Check sheet for the modelled part. Datum: model origin and axes. Units: mm. A direction names the side the tool comes from. Give positions to 0.01 mm unless a question says otherwise; leave off trailing zeros. Order: outer loops, then holes, each group sorted by start corner. A loop starts at its lowest first (then second) coordinate and runs counter-clockwise, first axis right, second up.
```python
from build123d import *

# Parameters (mm, degrees)
BOSS_EXTRUDE1_DEPTH     = 5.3
CIRPATTERN1_COUNT       = 10
FILLET1_R               = 0.2
FILLET3_R               = 0.2
SKETCH2_R               = 10
SKETCH2_R_2             = 4.05
BOSS_EXTRUDE2_DEPTH     = 16.7
CUT_EXTRUDE1_DEPTH      = 29.341701561
CUT_EXTRUDE1_DEPTH_BACK = 29.341701561
SKETCH2_2_R             = 4.05


with BuildPart() as part:
    # Sketch1 → Boss-Extrude1 (new body)
    with BuildSketch(Plane(origin=(0, 0, 0), x_dir=(0, 0, -1), z_dir=(1, 0, 0))):
        with BuildLine():
            Line((0, 0), (0, 16.75))
            Line((0, 16.75), (1.800167381, 14.035023954))
            ThreePointArc((1.800167381, 14.035023954), (3.754556482, 11.555336673), (6.793214092, 12.412684734))
            Line((6.793214092, 12.412684734), (9.845402976, 13.551034656))
            Line((9.845402976, 13.551034656), (0, 0))
        make_face()
    boss_extrude1 = extrude(amount=BOSS_EXTRUDE1_DEPTH)

    # CirPattern1: Boss-Extrude1 ×10 about axis
    cirpattern1_axis = Axis((0, 0, 0), (1, 0, 0))
    for i in range(1, CIRPATTERN1_COUNT):
        add(boss_extrude1.rotate(cirpattern1_axis, i * 360 / CIRPATTERN1_COUNT))

    # Fillet1
    fillet1_edges = [part.edges().sort_by_distance(p)[0] for p in [
        (2.65, 16.75, 0),
    ]]
    fillet(fillet1_edges, radius=FILLET1_R)

    # Fillet3
    fillet3_edges = [part.edges().sort_by_distance(p)[0] for p in [
        (2.65, 13.551034656, -9.845402976),
        (2.65, 13.551034656, 9.845402976),
        (2.65, 5.176034656, 15.930196648),
        (2.65, -5.176034656, 15.930196648),
        (2.65, -13.551034656, 9.845402976),
        (2.65, -16.75, 0),
        (2.65, -13.551034656, -9.845402976),
        (2.65, -5.176034656, -15.930196648),
        (2.65, 5.176034656, -15.930196648),
    ]]
    fillet(fillet3_edges, radius=FILLET3_R)

    # Sketch2 → Boss-Extrude2 (add)
    with BuildSketch(Plane.ZY):
        with Locations(Location((0, 0, 0), (0, 0, 180))):
            Circle(SKETCH2_R)
        Circle(SKETCH2_R_2, mode=Mode.SUBTRACT)
    extrude(amount=BOSS_EXTRUDE2_DEPTH)

    # Sketch2_2 → Cut-Extrude1 (cut, two sides: drawn at the far end of the back side and taken through both)
    with BuildSketch(Plane.ZY.offset(-CUT_EXTRUDE1_DEPTH_BACK)):
        Circle(SKETCH2_2_R)
    extrude(amount=CUT_EXTRUDE1_DEPTH + CUT_EXTRUDE1_DEPTH_BACK, mode=Mode.SUBTRACT)


solid = part.part
```
(1) Sectioned sample at B-B (z = -1). Enter the section's corners in (x, y).
(2) Thickness scan on L1, parallel to Y at x = -3, z = 0; L2, parallel to X at y = 6, z = 8.5; L3, parallel to Y at x = -15, z = 2. Record the ranges inside material, lowest first.
(3) Go/stop test with flat-tipped pins: P1, Ø2, axis at x = -13.5, y = -7, coming from the +Z side; P2, Ø12, axis at x = -7, y = 12, coming from the -Z side; P3, Ø4, axis at x = -9, z = -3, coming from the -Y side. Record where each tip stops, or that it passes through.
(4) Sectioned sample at A-A (y = 0). Enter the section's corners in (x, z), plus the area to 3 significant figures.
(5) Release check for a two-part mould opening along Y. For faces 1 (the face through (2.613, 12.922, -8.159)), 2 (the face through (2.613, -3.766, -14.811)), 3 (the face through (-16.7, -0.1, -4.3)) record: released by +Y, released by -Y, zero draft, split by the parting line, or undercut.
(6) Tool access check on faces 4 (the face through (2.613, 12.936, 8.197)), 5 (the face through (0, 2, -10)), 6 (the face through (2.61, -11.79, 9.77)), 7 (the face through (2.61, -11.75, -9.77)). Record the directions out of +Z, -Z, +X, -X, +Y, -Y that give a thin tool (end or side, any length) a straight path to the whole face; none if there is none.
(7) Sectioned sample at C-C (y = -12). Enter the section's corners in (x, z).
(8) Sectioned sample at D-D (x = -2.75). Enter the section's corners in (y, z).
Values follow:
1. outline: (-16.7, -9.95) - (0, -9.95) - (0, -15.24) - (5.3, -15.24) - (5.3, -3.92) - (-16.7, -3.92) - close; (-16.7, 3.92) - (5.3, 3.92) - (5.3, 15.24) - (0, 15.24) - (0, 9.95) - (-16.7, 9.95) - close
2. L1: y = -10 to -4.05, 4.05 to 10
2. L2: x = 0 to 5.3
2. L3: y = -9.8 to -3.52, 3.52 to 9.8
3. P1: stops at z = 8
3. P2: stops at z = -8
3. P3: stops at y = -9.95
4. outline: (-16.7, -10) - (0, -10) - (0, -12.15) - (5.3, -12.15) - (5.3, -4.05) - (-16.7, -4.05) - close; (-16.7, 4.05) - (5.3, 4.05) - (5.3, 12.15) - (0, 12.15) - (0, 10) - (-16.7, 10) - close
4. area: 285 mm2
5. face 1: released by +Y
5. face 2: undercut
5. face 3: zero draft
6. face 4: +X, -X, +Y
6. face 5: -X
6. face 6: +Z, +X, -X
6. face 7: -Z, +X, -X
7. outline: (0, -9.78) - (5.3, -9.78) - (5.3, -6.36) - (0, -6.36) - close; (0, -2.91) - (5.3, -2.91) - (5.3, 2.91) - (0, 2.91) - close; (0, 6.36) - (5.3, 6.36) - (5.3, 9.78) - (0, 9.78) - close
8. outline: circle Ø20 at (0, 0); hole circle Ø8.1 at (0, 0)
